Autodesk Inventor part; units mm, degrees
ref_plane "YZ Plane" through (0, 0, 0) normal (1, 0, 0) x (0, 1, 0)
ref_plane "XZ Plane" through (0, 0, 0) normal (0, 1, 0) x (-1, 0, 0)
ref_plane "XY Plane" through (0, 0, 0) normal (0, 0, 1) x (1, 0, 0)
sketch "Szkic1" plane through (0, 0, 0) normal (0, 1, 0) x (-1, 0, 0)
  line L0 (-2, 2) -> (2, 2)
  line L1 (2, 2) -> (2, -2)
  line L2 (2, -2) -> (-2, -2)
  line L3 (-2, -2) -> (-2, 2)
  line L4 (-2, 2) -> (2, -2) construction
  line L5 (2, 2) -> (-2, -2) construction
  point P0 (0, 0)
  dimension "d0" = 4
  dimension "d1" = 4
extrude "Wyciągnięcie proste1" add sketch "Szkic1" along normal blind 10
fillet "Zaokrąglenie1" radius 4 1 edges at (-2, 5, 2)
sketch "Szkic2" plane through (0, 10, 0) normal (0, 1, 0) x (1, 0, 0)
  circle A0 centre (0, 0) radius 1
  dimension "d5" = 2
extrude "Wyciągnięcie proste2" add sketch "Szkic2" along normal blind 2
properties part number "FanLegs"
Geometry: final body of the model. Coordinates: model frame, mm. A direction names the side the tool comes from. Round coordinates to 2 decimals unless told otherwise and drop trailing zeros. Order: outer loops, then holes, each group sorted by start corner. A loop starts at its lowest first (then second) coordinate and runs counter-clockwise, first axis right, second up. Notation, with made-up numbers: (67.5, 10) -> (115.5, 10) arc R26 ccw to (115.5, 29) -> close; hole circle Ø4 at (69, 24.25). An arc over 180 degrees is marked (long way). Use CSV: the item, a comma, the result in double quotes. Start each with the question number.
1) Section C-C (z = 0). Return the cut outline in (x, y).
2) First-contact query: pin 1 Ø1 at (x, y) = (0, 4.5) entering from +Z; pin 2 Ø2 at (y, z) = (8, -1) entering from -X. Flat tips, straight axial feed; report the tip coordinate or a pass-through.
3) Section B-B (x = 0). Return the cut outline in (y, z).
4) Material intervals for line 1 along Y through (x, z) = (0.9, 1.4); line 2 along X through (y, z) = (7.25, 0.3); line 3 along X through (y, z) = (1.25, -1.15), sorted ascending. Write a range as from..to.
5) Set-up query: faces 1 (the face through (1, 10, -1)), 2 (the face through (2, 5, 0)). Return all of +Z, -Z, +X, -X, +Y, -Y with unobstructed straight access to the full face (end or side cutting, diameter ignored); none if empty.
Returned:
1,outline,"(-1.46, 0) -> (2, 0) -> (2, 10) -> (1, 10) -> (1, 12) -> (-1, 12) -> (-1, 10) -> (-1.46, 10) -> close"
2,pin 1,"stops at z = 1.71"
2,pin 2,"stops at x = -2"
3,outline,"(0, -2) -> (10, -2) -> (10, -1) -> (12, -1) -> (12, 1) -> (10, 1) -> (10, 1.46) -> (0, 1.46) -> close"
4,line 1,"y = 0..10"
4,line 2,"x = -1.27..2"
4,line 3,"x = -1.91..2"
5,face 1,"+Y"
5,face 2,"+Z, -Z, +X, +Y, -Y"
